Can you work these out from the model? Positions are in its coordinate system, mm. A direction names the side the tool comes from. Coordinates: 2 decimals unless noted, no trailing zeros. Order: outer loops, then holes, each group sorted by start corner. A loop starts at its lowest first (then second) coordinate and runs counter-clockwise, first axis right, second up. Notation, with made-up numbers: (50.25, 14.25) -> (60.25, 14.25) arc R28 cw to (60.25, 52.25) -> close; hole circle Ø2 at (-31.5, 12.5). An arc over 180 degrees is marked (long way). Answer in a Markdown table with one row per item.
```python
from build123d import *

# Parameters (mm, degrees)
F0_W     = 6
F0_H     = 3
F0_R     = 1.75
F0_W_2   = 4
F1_DEPTH = 3


with BuildPart() as f1:
    # F0 (on Right) → F1 (new body)
    with BuildSketch(Plane.YZ):
        Polygon((6, -37), (6, 37), (2, 37), (-2, 37), (-6, 37), (-6, -37), (-2, -37), (2, -37), align=None)
        with Locations((0, -32.5)):
            Rectangle(F0_W, F0_H, mode=Mode.SUBTRACT)
        with Locations((0, -17)):
            Circle(F0_R, mode=Mode.SUBTRACT)
        with Locations((0, 17)):
            Circle(F0_R, mode=Mode.SUBTRACT)
        with Locations((0, 32.5)):
            Rectangle(F0_W, F0_H, mode=Mode.SUBTRACT)
        with Locations((4, 38.5)):
            Rectangle(F0_W_2, F0_H)
        with Locations((4, -38.5)):
            Rectangle(F0_W_2, F0_H)
        with Locations((-4, 38.5)):
            Rectangle(F0_W_2, F0_H)
        with Locations((-4, -38.5)):
            Rectangle(F0_W_2, F0_H)
    extrude(amount=F1_DEPTH)


solid = f1.part
```
(1) Suppose I cut it at A-A (y = 0). Please give me the cut outline in (x, z).
Response values:
| item | result |
|---|---|
| outline | (0, -37) -> (3, -37) -> (3, -34) -> (0, -34) -> close; (0, -31) -> (3, -31) -> (3, -18.75) -> (0, -18.75) -> close; (0, -15.25) -> (3, -15.25) -> (3, 15.25) -> (0, 15.25) -> close; (0, 18.75) -> (3, 18.75) -> (3, 31) -> (0, 31) -> close; (0, 34) -> (3, 34) -> (3, 37) -> (0, 37) -> close |
(2) We'd pull the mould along Y, two halves only. Please class faces 5 (the flat face through (1, 3, 32)), 6 (the flat face through (1, 6, -1)), 7 (the flat face through (1, -4, 40)): +Y half, -Y half, draft (parallel to the pull), parting line (faces both ways), or undercut.
Response values:
| item | result |
|---|---|
| face 5 | undercut |
| face 6 | +Y half |
| face 7 | draft |
(3) I need wall thicknesses on line 1 (Z direction, x = 1.4, y = 0); line 2 (Z direction, x = 1.35, y = 2.5); line 3 (Z direction, x = 0.35, y = -0.75). Which ranges of each line are inside material? Lowest first, please. Write a range as [from, to].
Response values:
| item | result |
|---|---|
| line 1 | [-37, -34], [-31, -18.75], [-15.25, 15.25], [18.75, 31], [34, 37] |
| line 2 | [-40, -34], [-31, 31], [34, 40] |
| line 3 | [-37, -34], [-31, -18.58], [-15.42, 15.42], [18.58, 31], [34, 37] |
(4) Will these pins go through, and if not, where does the flat tip stop? pin 1 Ø1.5 at (x, y) = (1, -1) entering from +Z; pin 2 Ø0.9 at (x, y) = (1.5, 1.5) entering from -Z.
Response values:
| item | result |
|---|---|
| pin 1 | z = 37 |
| pin 2 | z = -37 |
(5) Suppose I cut it at B-B (z = -17). Please give me the cut outline in (x, y).
Response values:
| item | result |
|---|---|
| outline | (0, -6) -> (3, -6) -> (3, -1.75) -> (0, -1.75) -> close; (0, 1.75) -> (3, 1.75) -> (3, 6) -> (0, 6) -> close |
(6) Suppose I cut it at C-C (x = 0.85). Please give me the cut outline in (y, z).
Response values:
| item | result |
|---|---|
| outline | (-6, -40) -> (-2, -40) -> (-2, -37) -> (2, -37) -> (2, -40) -> (6, -40) -> (6, 40) -> (2, 40) -> (2, 37) -> (-2, 37) -> (-2, 40) -> (-6, 40) -> close; hole (-3, -34) -> (3, -34) -> (3, -31) -> (-3, -31) -> close; hole (-3, 31) -> (3, 31) -> (3, 34) -> (-3, 34) -> close; hole circle Ø3.5 at (0, -17); hole circle Ø3.5 at (0, 17) |
(7) On a 3-axis mill with a long thin cutter (end or side, diameter ignored), from which of +Z, -Z, +X, -X, +Y, -Y can I reach the whole of each face in a straight line? I mean faces 1 (the flat face through (1, -2, 38)), 2 (the flat face through (1, -6, 1)), 3 (the flat face through (1, 0, -37)), 4 (the flat face through (1, 0, 34)). Say none if no direction works.
Response values:
| item | result |
|---|---|
| face 1 | +Z, +X, -X |
| face 2 | +Z, -Z, +X, -X, -Y |
| face 3 | -Z, +X, -X |
| face 4 | +X, -X |
